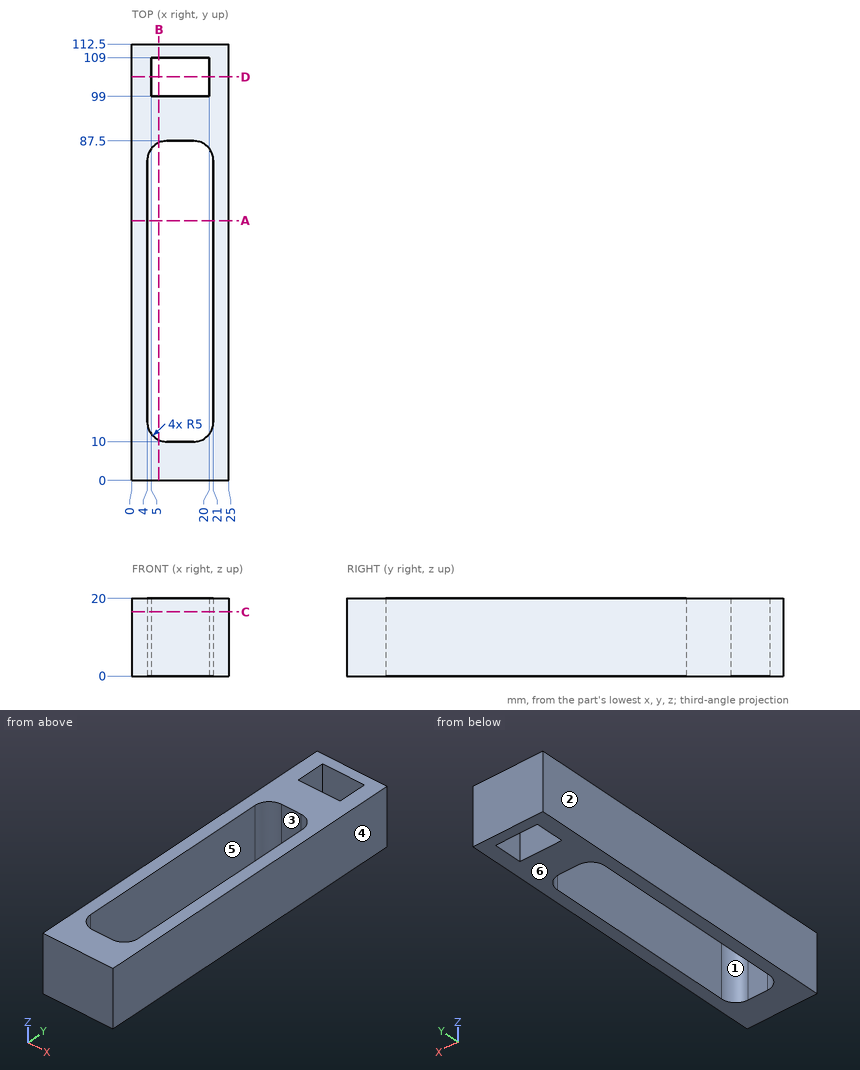
Source: three-view drawing plus pictorial views. Frame: mm from the lowest corner of the part. A direction names the side the tool comes from. Round coordinates to 2 decimals unless told otherwise and drop trailing zeros. Loops run counter-clockwise (first coordinate to the right, second up) from the corner with the lowest first, then second, coordinate; pieces in that order, holes last. Notation, with made-up numbers: M -35.5,78 L -30.5,78 A9 cw -30.5,95 Z; hole C 44.5,-17.75 d4. An arc over 180 degrees is marked long. Answer as CSV lines item,"result". Start each with the question number.
(1) Line query: line 1 (Y direction, x = 8.75, z = 6.75); line 2 (X direction, y = 15, z = 1); line 3 (Y direction, x = 17, z = 10). Output: solid intervals per line, ascending. Write a range as [from, to].
(2) Section D-D, the plane y = 104. Output: boundary loops of the cut face in (x, z), plus the area to 3 significant figures.
(3) Section C-C, the plane z = 16.5. Output: boundary loops of the cut face in (x, y), plus the area to 3 significant figures.
(4) Section A-A, the plane y = 67. Output: boundary loops of the cut face in (x, z), plus the area to 3 significant figures.
(5) Section B-B, the plane x = 7. Output: boundary loops of the cut face in (y, z).
(6) Draft query along X for the marked faces 3, 4, 5 and 6. Return one class per face: released by +X, released by -X, zero draft, split by the parting line, or undercut.
(7) Reachability of the marked faces 1 and 2 from +Z, -Z, +X, -X, +Y, -Y: full face, straight path, thin tool, end or side. Return the list, or none.
Values found:
1,line 1,"y = [0, 10.01], [87.49, 99], [109, 112.5]"
1,line 2,"x = [0, 4], [21, 25]"
1,line 3,"y = [0, 10.1], [87.4, 99], [109, 112.5]"
2,outline,"M 0,0 L 5,0 L 5,20 L 0,20 Z; M 20,0 L 25,0 L 25,20 L 20,20 Z"
2,area,"200 mm²"
3,outline,"M 0,0 L 25,0 L 25,112.5 L 0,112.5 Z; hole M 4,15 A5 ccw 9,10 L 16,10 A5 ccw 21,15 L 21,82.5 A5 ccw 16,87.5 L 9,87.5 A5 ccw 4,82.5 Z; hole M 5,99 L 20,99 L 20,109 L 5,109 Z"
3,area,"1,370 mm²"
4,outline,"M 0,0 L 4,0 L 4,20 L 0,20 Z; M 21,0 L 25,0 L 25,20 L 21,20 Z"
4,area,"160 mm²"
5,outline,"M 0,0 L 10.42,0 L 10.42,20 L 0,20 Z; M 87.08,0 L 99,0 L 99,20 L 87.08,20 Z; M 109,0 L 112.5,0 L 112.5,20 L 109,20 Z"
6,face 3,"undercut"
6,face 4,"released by +X"
6,face 5,"undercut"
6,face 6,"zero draft"
7,face 1,"+Z, -Z"
7,face 2,"+Z, -Z, -X, +Y, -Y"
